```python
from build123d import *

# Parameters (mm, degrees)
BOSS_EXTRUDE1_DEPTH     = 4.8
SKETCH3_R               = 2.675
BOSS_EXTRUDE2_DEPTH     = 28.7
FILLET1_R               = 0.25
CUT_EXTRUDE1_DEPTH      = 30.358769452
CUT_EXTRUDE1_DEPTH_BACK = 30.358769452
SKETCH4_W               = 15.294544115
SKETCH4_H               = 19.173595159


with BuildPart() as part:
    # Sketch2 → Boss-Extrude1 (new body)
    with BuildSketch(Plane(origin=(0, 0, 0), x_dir=(1, 0, 0), z_dir=(0, 1, 0))):
        Polygon((-2.3375, 4.048668763), (-4.675, 0), (-2.3375, -4.048668763), (2.3375, -4.048668763), (4.675, 0), (2.3375, 4.048668763), align=None)
    extrude(amount=BOSS_EXTRUDE1_DEPTH)

    # Sketch3 → Boss-Extrude2 (add)
    with BuildSketch(Plane.XZ):
        with Locations(Location((0, 0, 0), (0, 0, 270))):
            Circle(SKETCH3_R)
    extrude(amount=BOSS_EXTRUDE2_DEPTH)

    # Fillet1
    fillet1_edges = [part.edges().sort_by_distance(p)[0] for p in [
        (0, 0, 2.675),
    ]]
    fillet(fillet1_edges, radius=FILLET1_R)

    # Sketch4 → Cut-Extrude1 (cut, two sides: drawn at the far end of the back side and taken through both)
    with BuildSketch(Plane.XY.offset(-CUT_EXTRUDE1_DEPTH_BACK)):
        with Locations((0.498735134, -22.286797579)):
            Rectangle(SKETCH4_W, SKETCH4_H)
    extrude(amount=CUT_EXTRUDE1_DEPTH + CUT_EXTRUDE1_DEPTH_BACK, mode=Mode.SUBTRACT)


solid = part.part
```
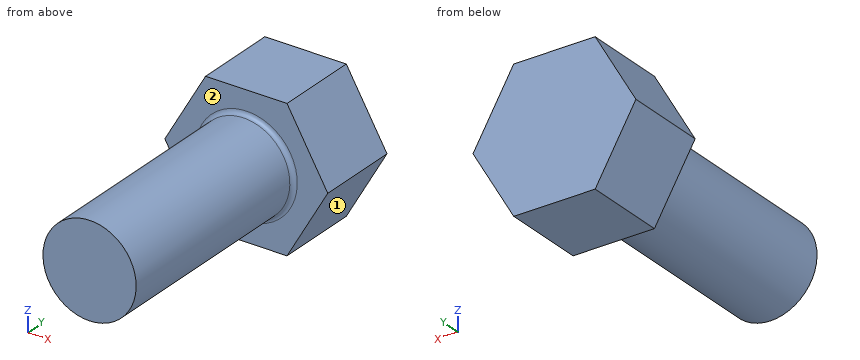
Here's how the part is built. I have some questions about the finished solid (model axes, mm). Face numbers are marked on the shaded views. A direction names the side the tool comes from. Round coordinates to 2 decimals unless told otherwise and drop trailing zeros. Write each loop counter-clockwise with the first axis right and the second up, starting at its lowest first coordinate (ties: lowest second). Pieces come first, ordered by that corner, then holes. Notation, with made-up numbers: M 34.25,14 L 48.25,14 A30 cw 48.25,52 Z; hole C -24,-33 d2. An arc over 180 degrees is marked long. Answer as CSV lines item,"result". Start each with the question number.
1. Suppose I cut it at B-B on y = 1.25. Write out the boundary of the cut face in (x, z) (1 decimal), then the cut area to 3 significant figures.
2. Suppose I cut it at C-C on z = -3.5. Write out the boundary of the cut face in (x, y).
3. On a 3-axis mill with a long thin cutter (end or side, diameter ignored), from which of +Z, -Z, +X, -X, +Y, -Y can I reach the whole of each face in a straight line? I mean the marked faces 1 and 2. Say none if no direction works.
4. Suppose I cut it at A-A on x = 0. Write out the boundary of the cut face in (y, z) (3 decimals).
5. I'm going to push flat-ended pins straight in: pin 1 Ø1 at (y, z) = (-1.5, -2.5) entering from -X; pin 2 Ø4 at (x, y) = (2, -3) entering from +Z (3 decimals); pin 3 Ø3 at (x, y) = (0, -3.5) entering from -Z (3 decimals). Where does each tip first touch, or does it pass through?
6. Suppose I cut it at D-D on y = -5.5. Write out the boundary of the cut face in (x, z) (3 decimals), then the cut area to 3 significant figures.
7. I need wall thicknesses on probe 1 along Y at (x, z) = (-2.75, -1.5); probe 2 along Z at (x, y) = (0, -5.75) (3 decimals); probe 3 along X at (y, z) = (-7.5, 0.25). Which ranges of each line are inside material? Lowest first, please.
Check result:
1,outline,"M -4.7,0 L -2.3,-4 L 2.3,-4 L 4.7,0 L 2.3,4 L -2.3,4 Z"
1,area,"56.8 mm2"
2,outline,"M -2.65,0 L 2.65,0 L 2.65,4.8 L -2.65,4.8 Z"
3,face 1,"-Z, +X, +Y, -Y"
3,face 2,"-Y"
4,outline,"M -12.7,-2.675 L -0.25,-2.675 A0.25 cw 0,-2.925 L 0,-4.049 L 4.8,-4.049 L 4.8,4.049 L 0,4.049 L 0,2.925 A0.25 cw -0.25,2.675 L -12.7,2.675 Z"
5,pin 1,"stops at x = -1.78"
5,pin 2,"stops at z = 2.675"
5,pin 3,"stops at z = -2.675"
6,outline,"C 0,0 d5.35"
6,area,"22.5 mm2"
7,probe 1,"y = 0 to 4.8"
7,probe 2,"z = -2.675 to 2.675"
7,probe 3,"x = -2.66 to 2.66"
